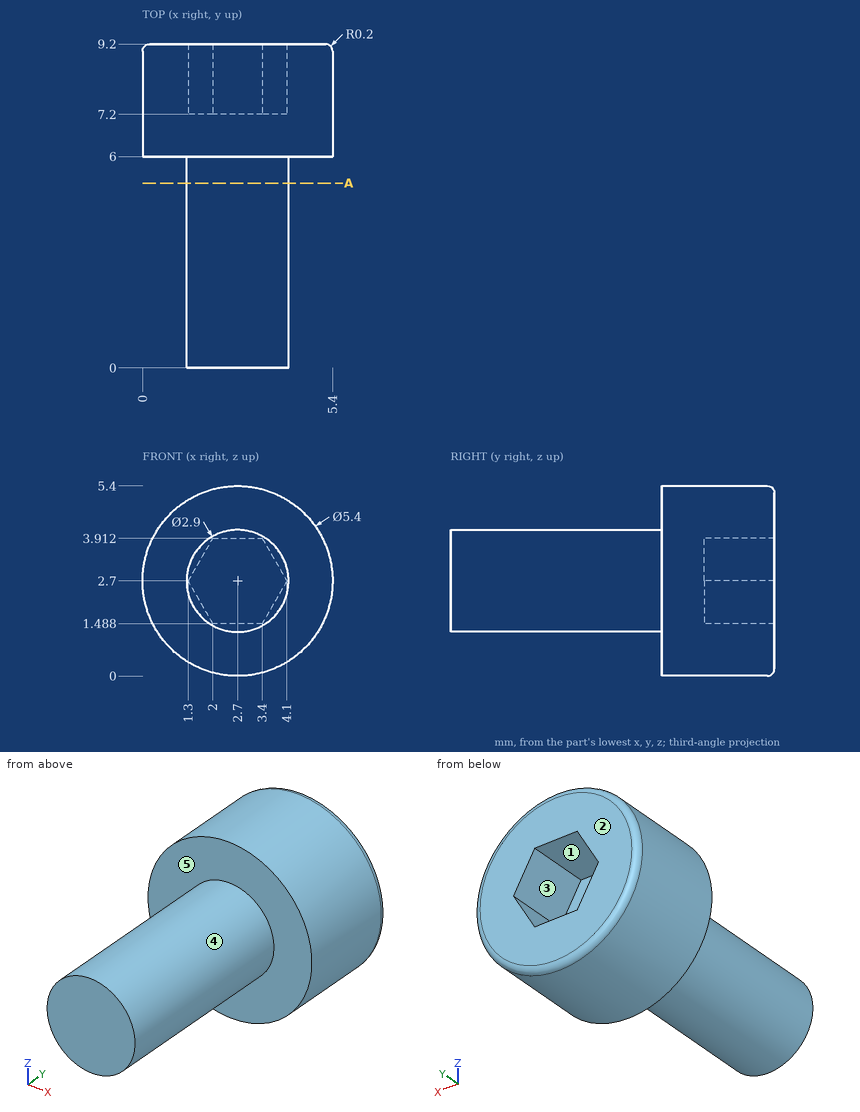
The drawing under review shows one solid part. Ordinate dimensions are in mm from its lowest x, y, z. A direction names the side the tool comes from. Round coordinates to 2 decimals unless told otherwise and drop trailing zeros. Write each loop counter-clockwise with the first axis right and the second up, starting at its lowest first coordinate (ties: lowest second). Pieces come first, ordered by that corner, then holes.
(1) Wall thickness on L1, parallel to Y at x = 3.75, z = 5; L2, parallel to Z at x = 3.2, y = 7.75; L3, parallel to Y at x = 1.95, z = 2.3: over which ranges is each line inside the solid? List them lowest first.
(2) Insertion check: pin 1 (1.5 mm diameter, centred on y = 1, z = 2.5, fed in from -X); pin 2 (3 mm diameter, centred on x = 1.5, y = 2, fed in from -Z). Each pin has a flat end and moves straight along its axis. Give the tip position at first contact, or say it passes through.
(3) Mouldability with a two-part tool opening along X and no side actions: class the marked faces 3, 4 and 5 as +X half, -X half, draft (parallel to the pull), parting line (faces both ways), or undercut.
(4) Machinability: for the marked faces 1 and 2, which of the approach directions +Z, -Z, +X, -X, +Y, -Y give a long, thin tool a straight path to every point of the face, cutting with its end or side? Answer none if there is none.
(5) We need section A-A on y = 5.25. Give the boundary of the cut face in (x, z).
Findings below:
1. L1: y = 6 to 9.2
1. L2: z = 0.05 to 1.49, 3.91 to 5.35
1. L3: y = 0 to 7.2
2. pin 1: stops at x = 1.25
2. pin 2: stops at z = 1.25
3. face 3: undercut
3. face 4: parting line
3. face 5: draft
4. face 1: +Y
4. face 2: +Z, -Z, +X, -X, +Y
5. outline: circle Ø2.9 at (2.7, 2.7)
